Check sheet for the drawn part. Datum: minimum x, y, z corner. Units: mm. A direction names the side the tool comes from. Round coordinates to 2 decimals unless told otherwise and drop trailing zeros. Order: outer loops, then holes, each group sorted by start corner. A loop starts at its lowest first (then second) coordinate and runs counter-clockwise, first axis right, second up. Notation, with made-up numbers: (-5, 18.5) -> (20, 18.5) arc R9 ccw to (20, 30.5) -> close; hole circle Ø7 at (-14, -27). An arc over 180 degrees is marked (long way). Answer as CSV lines item,"result". Start each with the question number.
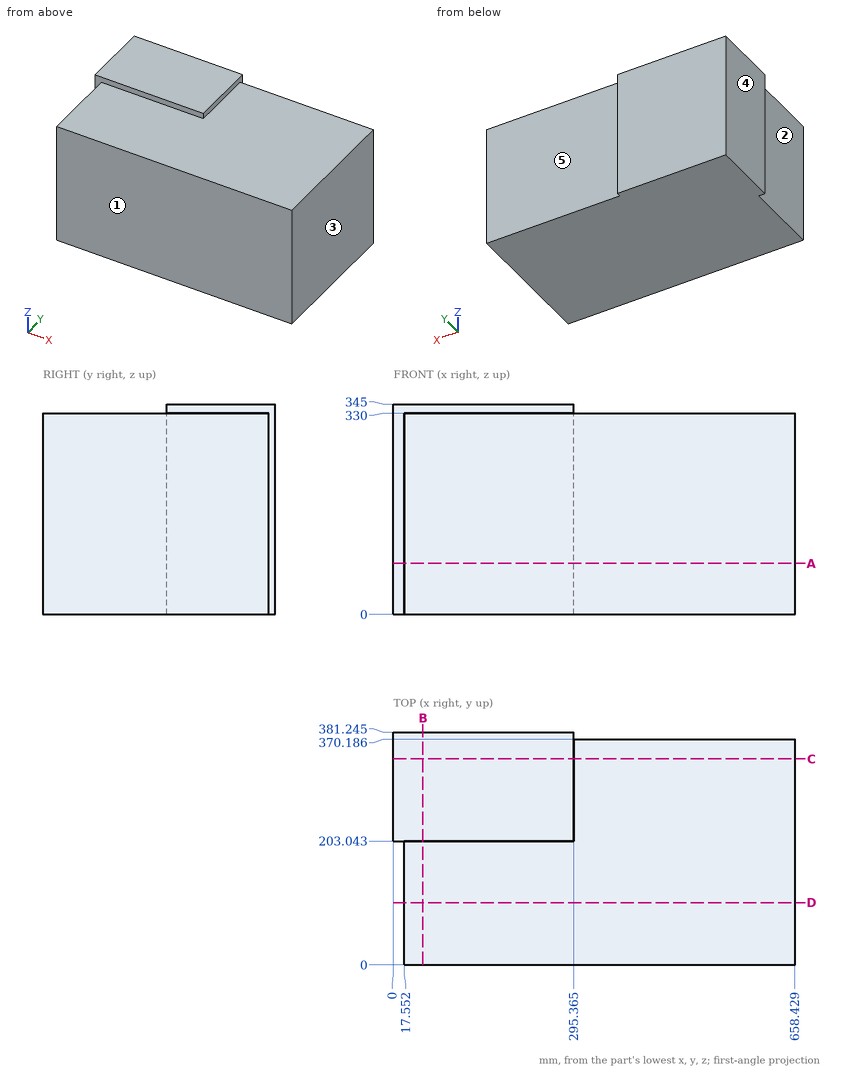
1) Section check D-D on y = 102. Record the cut outline in (x, z), then the cut area to 3 significant figures.
2) Access from +Z, -Z, +X, -X, +Y, -Y to the whole of each face (thin tool, end or side, straight path). Record for the marked faces 1 and 2.
3) Material ranges on line 1 along Z through (x, y) = (358, 43.5); line 2 along Y through (x, z) = (580.5, 250.5); line 3 along X through (y, z) = (123, 258), recorded low to high.
4) Section check B-B on x = 48. Record the cut outline in (y, z) (1 decimal), then the cut area to 3 significant figures.
5) Section check A-A on z = 83.5. Record the cut outline in (x, y) (1 decimal).
6) Mould release check, pull along X, two halves, no side actions. Record for the marked faces 3, 4 and 5: released by +X, released by -X, zero draft, split by the parting line, or undercut.
7) Section check C-C on y = 338. Record the cut outline in (x, z) (1 decimal).
8) Depth check by flat-ended pin: pin 1 Ø1 at (y, z) = (75, 173) entering from -X; pin 2 Ø2 at (x, z) = (553.5, 60.5) entering from -Y; pin 3 Ø1 at (x, y) = (510.5, 291) entering from +Z; pin 4 Ø4 at (x, z) = (300.5, 208) entering from +Y. Enter the tip coordinate at first touch or a pass-through.
Solutions:
1,outline,"(17.55, 0) -> (658.43, 0) -> (658.43, 330) -> (17.55, 330) -> close"
1,area,"211,000 mm^2"
2,face 1,"+Z, -Z, +X, -X, -Y"
2,face 2,"+Z, -Z, -X, -Y"
3,line 1,"z = 0 to 330"
3,line 2,"y = 0 to 370.19"
3,line 3,"x = 17.55 to 658.43"
4,outline,"(0, 0) -> (381.2, 0) -> (381.2, 345) -> (203, 345) -> (203, 330) -> (0, 330) -> close"
4,area,"128,000 mm^2"
5,outline,"(0, 203) -> (17.6, 203) -> (17.6, 0) -> (658.4, 0) -> (658.4, 370.2) -> (295.4, 370.2) -> (295.4, 381.2) -> (0, 381.2) -> close"
6,face 3,"released by +X"
6,face 4,"released by -X"
6,face 5,"zero draft"
7,outline,"(0, 0) -> (658.4, 0) -> (658.4, 330) -> (295.4, 330) -> (295.4, 345) -> (0, 345) -> close"
8,pin 1,"stops at x = 17.55"
8,pin 2,"stops at y = 0"
8,pin 3,"stops at z = 330"
8,pin 4,"stops at y = 370.19"
